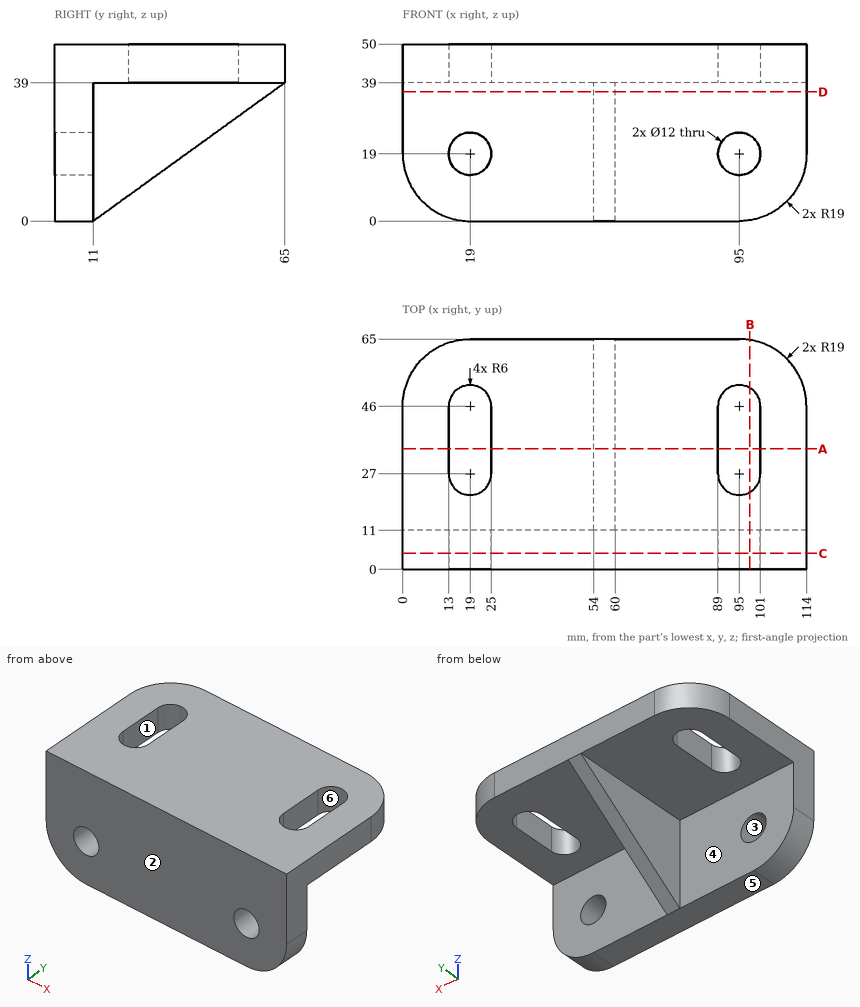
Study the drawing (mm; zero at the part's minimum x, y, z) and answer. A direction names the side the tool comes from. Give positions to 0.01 mm unless a question says otherwise; leave off trailing zeros. Write each loop counter-clockwise with the first axis right and the second up, starting at its lowest first coordinate (ties: lowest second). Pieces come first, ordered by that corner, then holes. Notation, with made-up numbers: (73, 0) -> (125, 0) arc R20 ccw to (125, 12) -> close; hole circle Ø8 at (79.25, -15). An arc over 180 degrees is marked (long way). Answer in a Markdown table with one row per item.
1) Determine the mould class of the marked faces 1, 2 and 3 for opening direction Y: released by +Y, released by -Y, zero draft, split by the parting line, or undercut.
Results list:
| item | result |
|---|---|
| face 1 | undercut |
| face 2 | released by -Y |
| face 3 | zero draft |
2) Each of these flat-tipped pins is pushed along its axis until it touches: pin 1 Ø12 at (x, z) = (26.5, 5.5) entering from -Y; pin 2 Ø8 at (y, z) = (7.5, 9) entering from -X; pin 3 Ø3 at (x, y) = (88.5, 40.5) entering from -Z; pin 4 Ø6 at (x, z) = (70, 5.5) entering from +Y. Where does it stop, or does it pass through?
Results list:
| item | result |
|---|---|
| pin 1 | y = 0 |
| pin 2 | x = 0.97 |
| pin 3 | z = 39 |
| pin 4 | y = 11 |
3) Section B-B on x = 98 is taken. Give the vertices of the cut face in (y, z), plus the area to 3 significant figures.
Results list:
| item | result |
|---|---|
| outline | (0, 0.24) -> (11, 0.24) -> (11, 13.8) -> (0, 13.8) -> close; (0, 24.2) -> (11, 24.2) -> (11, 39) -> (21.8, 39) -> (21.8, 50) -> (0, 50) -> close; (51.2, 39) -> (64.76, 39) -> (64.76, 50) -> (51.2, 50) -> close |
| area | 701 mm^2 |
4) Straight lines are drawn through the part: line 1 (X direction, y = 28.5, z = 43); line 2 (Z direction, x = 19, y = 4.75); line 3 (Y direction, x = 85.5, z = 35.5). For each, find the intervals that lie inside material, in ascending order. Write a range as [from, to].
Results list:
| item | result |
|---|---|
| line 1 | [0, 13], [25, 89], [101, 114] |
| line 2 | [0, 13], [25, 50] |
| line 3 | [0, 11] |
5) Section D-D on z = 36.5 is taken. Give the vertices of the cut face in (x, y), plus the area to 3 significant figures.
Results list:
| item | result |
|---|---|
| outline | (0, 0) -> (114, 0) -> (114, 11) -> (60, 11) -> (60, 61.54) -> (54, 61.54) -> (54, 11) -> (0, 11) -> close |
| area | 1,560 mm^2 |
6) Section A-A on y = 34 is taken. Give the vertices of the cut face in (x, z).
Results list:
| item | result |
|---|---|
| outline | (0, 39) -> (13, 39) -> (13, 50) -> (0, 50) -> close; (25, 39) -> (54, 39) -> (54, 16.61) -> (60, 16.61) -> (60, 39) -> (89, 39) -> (89, 50) -> (25, 50) -> close; (101, 39) -> (114, 39) -> (114, 50) -> (101, 50) -> close |
7) Section C-C on y = 4.5 is taken. Give the vertices of the cut face in (x, z).
Results list:
| item | result |
|---|---|
| outline | (0, 19) arc R19 ccw to (19, 0) -> (95, 0) arc R19 ccw to (114, 19) -> (114, 50) -> (0, 50) -> close; hole circle Ø12 at (19, 19); hole circle Ø12 at (95, 19) |
8) A tool of negligible diameter and unlimited length cuts with its end or side. For the marked faces 4, 5 and 6, from which of +Z, -Z, +X, -X, +Y, -Y can it reach the whole face along a straight path? Write none if from no direction.
Results list:
| item | result |
|---|---|
| face 4 | -Z, -X, +Y |
| face 5 | -Z, +X, -X, +Y, -Y |
| face 6 | +Z, -Z |
